Autodesk Inventor part; units mm, degrees
ref_plane "YZ Plane" through (0, 0, 0) normal (1, 0, 0) x (0, 1, 0)
ref_plane "XZ Plane" through (0, 0, 0) normal (0, 1, 0) x (-1, 0, 0)
ref_plane "XY Plane" through (0, 0, 0) normal (0, 0, 1) x (1, 0, 0)
sketch "Sketch1" plane through (0, 0, 0) normal (0, 1, 0) x (-1, 0, 0)
  line L0 (23.0187, -23.0187) -> (-23.0187, -23.0187)
  line L1 (-23.0187, -23.0187) -> (-23.0187, 23.0187)
  line L2 (-23.0187, 23.0187) -> (23.0187, 23.0187)
  line L3 (23.0187, 23.0187) -> (23.0187, -23.0187)
  line L4 (23.0187, -23.0187) -> (-23.0187, 23.0187) construction
  line L5 (-23.0187, -23.0187) -> (23.0187, 23.0187) construction
  line L6 (9.525, -14.2875) -> (-9.525, -14.2875) construction
  line L7 (9.525, -11.9062) -> (-9.525, -11.9062)
  line L8 (-9.525, -16.6688) -> (9.525, -16.6688)
  arc A0 (9.525, -16.6688) -> (9.525, -11.9062) centre (9.525, -14.2875) ccw
  arc A1 (-9.525, -11.9062) -> (-9.525, -16.6688) centre (-9.525, -14.2875) ccw
  line L9 (0, -32.2263) -> (0, 32.2263) construction
  line L10 (32.2263, 0) -> (-32.2263, 0) construction
  line L11 (9.525, 14.2875) -> (-9.525, 14.2875) construction
  line L12 (9.525, 11.9062) -> (-9.525, 11.9062)
  line L13 (-9.525, 16.6688) -> (9.525, 16.6688)
  arc A2 (9.525, 11.9062) -> (9.525, 16.6688) centre (9.525, 14.2875) ccw
  arc A3 (-9.525, 16.6688) -> (-9.525, 11.9062) centre (-9.525, 14.2875) ccw
  point P0 (0, 0)
  point P1 (0, -14.2875)
  point P2 (0, 14.2875)
  dimension "d0" = 46.0375
  dimension "d1" = 46.0375
  dimension "d2" = 19.05
  dimension "d3" = 4.7625
  dimension "d4" = 11.9062
  dimension "d5" = 11.9062
extrude "Extrusion1" add sketch "Sketch1" along normal blind 3.175
sketch "Sketch2" plane through (0, 3.175, 0) normal (0, 1, 0) x (1, 0, 0)
  line L0 (-23.0187, -23.0187) -> (23.0187, -23.0187) construction
  line L1 (23.0187, -23.0187) -> (23.0187, 23.0187) construction
  line L2 (23.0187, 23.0187) -> (-23.0187, 23.0187) construction
  line L3 (-23.0187, 23.0187) -> (-23.0187, -23.0187) construction
  line L4 (9.525, 11.9062) -> (-9.525, 11.9062) construction
  arc A0 (-9.525, 16.6688) -> (-9.525, 11.9062) centre (-9.525, 14.2875) ccw construction
  line L5 (-9.525, 16.6688) -> (9.525, 16.6688) construction
  arc A1 (9.525, 11.9062) -> (9.525, 16.6688) centre (9.525, 14.2875) ccw construction
  line L6 (9.525, -16.6688) -> (-9.525, -16.6688) construction
  arc A2 (-9.525, -11.9062) -> (-9.525, -16.6688) centre (-9.525, -14.2875) ccw construction
  line L7 (-9.525, -11.9062) -> (9.525, -11.9062) construction
  arc A3 (9.525, -16.6688) -> (9.525, -11.9062) centre (9.525, -14.2875) ccw construction
  circle A4 centre (0, 0) radius 9.525 construction
  line L8 (0, 32.2263) -> (0, -32.2263) construction
  point P0 (0, 9.525)
  dimension "d8" = 19.05
hole "Hole1" at (0, 3.175, -9.525) direction (0, -1, 0) diameter 2.2606 end through all
pattern_circular "Circular Pattern1" count 6 over 360 about axis through (0, -10, 0) along (0, 1, 0) of "Hole1"
sketch "Sketch4" plane through (0, 3.175, 0) normal (0, 1, 0) x (1, 0, 0)
  circle A0 centre (-19.05, 19.05) radius 1.7272
  circle A1 centre (19.05, 19.05) radius 1.7272
  circle A2 centre (8.2489, 4.7625) radius 1.1303 construction
  circle A3 centre (8.2489, -4.7625) radius 1.1303 construction
  circle A4 centre (0, -9.525) radius 1.1303 construction
  circle A5 centre (-8.2489, -4.7625) radius 1.1303 construction
  circle A6 centre (-8.2489, 4.7625) radius 1.1303 construction
  circle A7 centre (0, 9.525) radius 1.1303 construction
  line L0 (-23.0187, -23.0187) -> (23.0187, -23.0187) construction
  line L1 (23.0187, -23.0187) -> (23.0187, 23.0187) construction
  line L2 (23.0187, 23.0187) -> (-23.0187, 23.0187) construction
  line L3 (-23.0187, 23.0187) -> (-23.0187, -23.0187) construction
  line L4 (9.525, 11.9062) -> (-9.525, 11.9062) construction
  arc A8 (-9.525, 16.6688) -> (-9.525, 11.9062) centre (-9.525, 14.2875) ccw construction
  line L5 (-9.525, 16.6688) -> (9.525, 16.6688) construction
  arc A9 (9.525, 11.9062) -> (9.525, 16.6688) centre (9.525, 14.2875) ccw construction
  line L6 (9.525, -16.6688) -> (-9.525, -16.6688) construction
  arc A10 (-9.525, -11.9062) -> (-9.525, -16.6688) centre (-9.525, -14.2875) ccw construction
  line L7 (-9.525, -11.9062) -> (9.525, -11.9062) construction
  arc A11 (9.525, -16.6688) -> (9.525, -11.9062) centre (9.525, -14.2875) ccw construction
  line L8 (0, 32.2263) -> (0, -32.2263) construction
  line L9 (-32.2263, 0) -> (32.2263, 0) construction
  circle A12 centre (-19.05, -19.05) radius 1.7272
  circle A13 centre (19.05, -19.05) radius 1.7272
  point P0 (0, 0)
  dimension "d19" = 3.4544
  dimension "d20" = 38.1
  dimension "d21" = 19.05
  dimension "d22" = 38.1
  dimension "d23" = 38.1
extrude "Extrusion2" cut sketch "Sketch4" against normal blind 3.175
sketch "Sketch5" plane through (0, 3.175, 0) normal (0, 1, 0) x (1, 0, 0)
  circle A0 centre (-19.05, -19.05) radius 1.7272 construction
  circle A1 centre (19.05, 19.05) radius 1.7272 construction
  circle A2 centre (19.05, -19.05) radius 1.7272 construction
  circle A3 centre (-19.05, 19.05) radius 1.7272 construction
  circle A4 centre (8.2489, 4.7625) radius 1.1303 construction
  circle A5 centre (8.2489, -4.7625) radius 1.1303 construction
  circle A6 centre (0, -9.525) radius 1.1303 construction
  circle A7 centre (-8.2489, -4.7625) radius 1.1303 construction
  circle A8 centre (-8.2489, 4.7625) radius 1.1303 construction
  circle A9 centre (0, 9.525) radius 1.1303 construction
  line L0 (-23.0187, -23.0187) -> (23.0187, -23.0187) construction
  line L1 (23.0187, -23.0187) -> (23.0187, 23.0187) construction
  line L2 (23.0187, 23.0187) -> (-23.0187, 23.0187) construction
  line L3 (-23.0187, 23.0187) -> (-23.0187, -23.0187) construction
  line L4 (9.525, 11.9062) -> (-9.525, 11.9062) construction
  arc A10 (-9.525, 16.6688) -> (-9.525, 11.9062) centre (-9.525, 14.2875) ccw construction
  line L5 (-9.525, 16.6688) -> (9.525, 16.6688) construction
  arc A11 (9.525, 11.9062) -> (9.525, 16.6688) centre (9.525, 14.2875) ccw construction
  line L6 (9.525, -16.6688) -> (-9.525, -16.6688) construction
  arc A12 (-9.525, -11.9062) -> (-9.525, -16.6688) centre (-9.525, -14.2875) ccw construction
  line L7 (-9.525, -11.9062) -> (9.525, -11.9062) construction
  arc A13 (9.525, -16.6688) -> (9.525, -11.9062) centre (9.525, -14.2875) ccw construction
  line L8 (-32.2263, 0) -> (32.2263, 0) construction
  line L9 (0, 32.2263) -> (0, -32.2263) construction
  circle A14 centre (19.05, -19.05) radius 1.7272 construction
  line L10 (19.05, 19.05) -> (19.05, -19.05) construction
  point P0 (0, 0)
  point P1 (19.05, 4.7625)
  point P2 (19.05, -4.7625)
  dimension "d26" = 9.525
  dimension "d27" = 4.7625
hole "Hole2" at (19.05, 3.175, -4.7625) at (19.05, 3.175, 4.7625) direction (0, -1, 0) diameter 1.6942 end through all
equation "\"d21\" = 0.5 * d20"
properties part number "Table"
The model under review builds one solid part; all positions refer to its coordinate system, in mm. A direction names the side the tool comes from. Round coordinates to 2 decimals unless told otherwise and drop trailing zeros. Order: outer loops, then holes, each group sorted by start corner. A loop starts at its lowest first (then second) coordinate and runs counter-clockwise, first axis right, second up. Notation, with made-up numbers: (69, -37.5) - (108, -37.5) arc R33 ccw to (108, -0.5) - close; hole circle Ø10 at (84, -27.5). An arc over 180 degrees is marked (long way). Answer in a Markdown table with one row per item.
(1) Clearance check with a flat-ended pin moving along its axis: P1, Ø2.5, axis at x = 8.25, z = -4.76, coming from the -Y side. State where the tip first meets the part, or that it passes through.
Result set:
| item | result |
|---|---|
| P1 | stops at y = 0 |
(2) Machinability: for faces 1 (the face through (0, 0, 0)), 2 (the face through (0, 2, -16.669)), which of the approach directions +Z, -Z, +X, -X, +Y, -Y give a long, thin tool a straight path to every point of the face, cutting with its end or side? Answer none if there is none.
Result set:
| item | result |
|---|---|
| face 1 | +Z, -Z, +X, -X, -Y |
| face 2 | +Y, -Y |
(3) Take a section at A-A on x = -2. Write out the cut boundary in (y, z) (3 decimals).
Result set:
| item | result |
|---|---|
| outline | (0, -23.019) - (3.175, -23.019) - (3.175, -16.669) - (0, -16.669) - close; (0, -11.906) - (3.175, -11.906) - (3.175, 11.906) - (0, 11.906) - close; (0, 16.669) - (3.175, 16.669) - (3.175, 23.019) - (0, 23.019) - close |
(4) Take a section at B-B on z = 19.05. Write out the cut boundary in (x, y) (3 decimals).
Result set:
| item | result |
|---|---|
| outline | (-23.019, 0) - (-20.777, 0) - (-20.777, 3.175) - (-23.019, 3.175) - close; (-17.323, 0) - (17.323, 0) - (17.323, 3.175) - (-17.323, 3.175) - close; (20.777, 0) - (23.019, 0) - (23.019, 3.175) - (20.777, 3.175) - close |
(5) For line 1 (Z direction, x = 19.05, y = 1.2); line 2 (X direction, y = 1.5, z = -19); line 3 (Z direction, x = 5, y = 0.9), list the stretches that pass through material, from the lowest coordinate up. Write a range as from..to.
Result set:
| item | result |
|---|---|
| line 1 | z = -23.02..-20.78, -17.32..-5.61, -3.92..3.92, 5.61..17.32, 20.78..23.02 |
| line 2 | x = -23.02..-20.78, -17.32..17.32, 20.78..23.02 |
| line 3 | z = -23.02..-16.67, -11.91..11.91, 16.67..23.02 |
(6) Take a section at D-D on z = -15.5. Write out the cut boundary in (x, y) (1 decimal).
Result set:
| item | result |
|---|---|
| outline | (-23, 0) - (-11.6, 0) - (-11.6, 3.2) - (-23, 3.2) - close; (11.6, 0) - (23, 0) - (23, 3.2) - (11.6, 3.2) - close |
(7) Take a section at C-C on x = 19.05. Write out the cut boundary in (y, z) (3 decimals).
Result set:
| item | result |
|---|---|
| outline | (0, -23.019) - (3.175, -23.019) - (3.175, -20.777) - (0, -20.777) - close; (0, -17.323) - (3.175, -17.323) - (3.175, -5.61) - (0, -5.61) - close; (0, -3.915) - (3.175, -3.915) - (3.175, 3.915) - (0, 3.915) - close; (0, 5.61) - (3.175, 5.61) - (3.175, 17.323) - (0, 17.323) - close; (0, 20.777) - (3.175, 20.777) - (3.175, 23.019) - (0, 23.019) - close |
(8) Mouldability with a two-part tool opening along X and no side actions: class faces 3 (the face through (23.019, 2, 0)), 4 (the face through (7.8, 1.6, -5.8)), 5 (the face through (0, 2, -23.019)) as released by +X, released by -X, zero draft, split by the parting line, or undercut.
Result set:
| item | result |
|---|---|
| face 3 | released by +X |
| face 4 | undercut |
| face 5 | zero draft |
